```python
from build123d import *

# Parameters (mm, degrees)
SKETCH4_W           = 50
SKETCH4_H           = 60
BOSS_EXTRUDE6_DEPTH = 40
SKETCH9_W           = 42
SKETCH9_H           = 56.420845642
CUT_EXTRUDE3_DEPTH  = 60
SKETCH10_W          = 40
SKETCH10_H          = 20
CUT_EXTRUDE4_DEPTH  = 20
SKETCH11_R          = 5
CUT_EXTRUDE5_DEPTH  = 10


with BuildPart() as part:
    # Sketch4 → Boss-Extrude6 (new body)
    with BuildSketch(Plane(origin=(0, 0, 0), x_dir=(1, 0, 0), z_dir=(0, 1, 0))):
        Rectangle(SKETCH4_W, SKETCH4_H)
    extrude(amount=BOSS_EXTRUDE6_DEPTH)

    # Sketch9 → Cut-Extrude3 (cut)
    with BuildSketch(Plane.XY.offset(30)):
        with Locations((0, 38.210422821)):
            Rectangle(SKETCH9_W, SKETCH9_H)
    extrude(amount=-CUT_EXTRUDE3_DEPTH, mode=Mode.SUBTRACT)

    # Sketch10 → Cut-Extrude4 (cut)
    with BuildSketch(Plane(origin=(25, 0, 0), x_dir=(0, 0, -1), z_dir=(1, 0, 0))):
        with Locations((0, 20)):
            Rectangle(SKETCH10_W, SKETCH10_H)
    extrude(amount=-CUT_EXTRUDE4_DEPTH, mode=Mode.SUBTRACT)

    # Sketch11 → Cut-Extrude5 (cut)
    with BuildSketch(Plane.ZY.offset(25)):
        with Locations((-9.5, 20)):
            Circle(SKETCH11_R)
    extrude(amount=-CUT_EXTRUDE5_DEPTH, mode=Mode.SUBTRACT)


solid = part.part
```
The listing builds one solid part. Answer for the finished solid, in the listing's coordinates (mm). A direction names the side the tool comes from. Give positions to 0.01 mm unless a question says otherwise; leave off trailing zeros. Order: outer loops, then holes, each group sorted by start corner. A loop starts at its lowest first (then second) coordinate and runs counter-clockwise, first axis right, second up.
1) Find section B-B on y = 31.5. Write down the section's boundary in (x, z).
Reported:
outline: (-25, -30) - (-21, -30) - (-21, 30) - (-25, 30) - close; (21, -30) - (25, -30) - (25, 30) - (21, 30) - close
2) For faces 1 (the face through (23, 30, 0)), 2 (the face through (-21, 25, 0)), 3 (the face through (25, 6, 0)), determine the directions among +Z, -Z, +X, -X, +Y, -Y from which every point of the face is accessible in a straight line to the end or side of a thin tool.
Reported:
face 1: +X
face 2: +Z, -Z, +Y
face 3: +Z, -Z, +X, +Y, -Y
3) Find section C-C on z = -9.5. Write down the section's boundary in (x, y), then the cut area to 3 significant figures.
Reported:
outline: (-25, 0) - (25, 0) - (25, 10) - (-21, 10) - (-21, 15) - (-25, 15) - close; (-25, 25) - (-21, 25) - (-21, 40) - (-25, 40) - close; (21, 30) - (25, 30) - (25, 40) - (21, 40) - close
area: 620 mm2
4) Determine the mould class of faces 4 (the face through (-23, 40, 0)), 5 (the face through (23, 20, -20)), 6 (the face through (-25, 20, 0)) for opening direction Y: pulls with the +Y half, pulls with the -Y half, needs draft (parallel to the pull), parting line crosses it, or undercut.
Reported:
face 4: pulls with the +Y half
face 5: undercut
face 6: needs draft
5) Find section A-A on z = 7.5. Write down the section's boundary in (x, y), then the cut area to 3 significant figures.
Reported:
outline: (-25, 0) - (25, 0) - (25, 10) - (-21, 10) - (-21, 40) - (-25, 40) - close; (21, 30) - (25, 30) - (25, 40) - (21, 40) - close
area: 660 mm2
6) Find section D-D on y = 20. Write down the section's boundary in (x, z).
Reported:
outline: (-25, -30) - (-21, -30) - (-21, -14.5) - (-25, -14.5) - close; (-25, -4.5) - (-21, -4.5) - (-21, 30) - (-25, 30) - close; (21, -30) - (25, -30) - (25, -20) - (21, -20) - close; (21, 20) - (25, 20) - (25, 30) - (21, 30) - close
7) Given P1, Ø4, axis at y = 16, z = -7.5, coming from the +X side, flat-ended and moving along its own axis, determine where the tip first touches the part or whether it passes through.
Reported:
P1: stops at x = -21
8) Consider line 1 along X through (y, z) = (37.5, 21); line 2 along Y through (x, z) = (-23.45, -9.5); line 3 along Y through (x, z) = (22, 11.5). Determine where each line is inside the solid, lowest interval first.
Reported:
line 1: x = -25 to -21, 21 to 25
line 2: y = 0 to 15, 25 to 40
line 3: y = 0 to 10, 30 to 40
